Geometry check sheet. Reference: the model listing, model coordinates, mm. Face numbers are marked on the shaded views. A direction names the side the tool comes from. Round coordinates to 2 decimals unless told otherwise and drop trailing zeros. Write each loop counter-clockwise with the first axis right and the second up, starting at its lowest first coordinate (ties: lowest second). Pieces come first, ordered by that corner, then holes. Notation, with made-up numbers: M 33.5,37.5 L 46.5,37.5 A25 cw 46.5,65.5 Z; hole C 38,-36.75 d8. An arc over 180 degrees is marked long. Answer in a Markdown table with one row per item. Add a question column.
from build123d import *

# Parameters (mm, degrees)
EXTRUDE_1_DEPTH          = 0.75
PATTERN_CIRCULAR_1_COUNT = 14
SKETCH_3_W               = 6.1
SKETCH_3_H               = 6.1
EXTRUDE_2_DEPTH          = 9
FILLET_1_R               = 2
CHAMFER_1_SIZE           = 0.2
CHAMFER_1_SIZE2          = 2.286010461


with BuildPart() as part:
    # Sketch 1 → Revolve 1 (revolve)
    with BuildSketch(Plane(origin=(0, 0, 0), x_dir=(0, 0, -1), z_dir=(1, 0, 0)), mode=Mode.PRIVATE) as revolve_1_sk:
        Polygon((-5, 0), (5, 0), (5, 15), (3, 15), (3, 10), (-3, 10), (-3, 15), (-5, 15), align=None)
    revolve(revolve_1_sk.sketch.rotate(Axis((0, 0, 5), (0, 0, -1)), 90), axis=Axis((0, 0, 5), (0, 0, -1)))

    # Sketch 2 → Extrude 1 (add, symmetric)
    with BuildSketch(Plane(origin=(0, 0, 0), x_dir=(0, 0, -1), z_dir=(1, 0, 0))):
        with BuildLine():
            Line((3, 10), (3, 14))
            Line((3, 14), (2, 14))
            ThreePointArc((2, 14), (0, 12), (-2, 14))
            Line((-2, 14), (-3, 14))
            Line((-3, 14), (-3, 10))
            Line((-3, 10), (-3, 8.5))
            Line((-3, 8.5), (3, 8.5))
            Line((3, 8.5), (3, 10))
        make_face()
    extrude_1 = extrude(amount=EXTRUDE_1_DEPTH, both=True)

    # Pattern Circular 1: Extrude 1 ×14 about axis
    pattern_circular_1_axis = Axis((0, 0, 0), (0, 0, 1))
    for i in range(1, PATTERN_CIRCULAR_1_COUNT):
        add(extrude_1.rotate(pattern_circular_1_axis, i * 360 / PATTERN_CIRCULAR_1_COUNT))

    # Sketch 3 → Extrude 2 (add)
    with BuildSketch(Plane(origin=(0, 0, -5), x_dir=(-1, 0, 0), z_dir=(0, 0, -1))):
        with BuildLine():
            Line((-4.05, -6.05), (4.05, -6.05))
            ThreePointArc((4.05, -6.05), (5.464213562, -5.464213562), (6.05, -4.05))
            Line((6.05, -4.05), (6.05, 4.05))
            ThreePointArc((6.05, 4.05), (5.464213562, 5.464213562), (4.05, 6.05))
            Line((4.05, 6.05), (-4.05, 6.05))
            ThreePointArc((-4.05, 6.05), (-5.464213562, 5.464213562), (-6.05, 4.05))
            Line((-6.05, 4.05), (-6.05, -4.05))
            ThreePointArc((-6.05, -4.05), (-5.464213562, -5.464213562), (-4.05, -6.05))
        make_face()
        Rectangle(SKETCH_3_W, SKETCH_3_H, mode=Mode.SUBTRACT)
    extrude(amount=EXTRUDE_2_DEPTH)

    # Fillet 1
    fillet_1_edges = [part.edges().sort_by_distance(p)[0] for p in [
        (5.464213562, -5.464213562, -5),
        (0, -6.05, -5),
        (-5.464213562, -5.464213562, -5),
        (-6.05, 0, -5),
        (-5.464213562, 5.464213562, -5),
        (0, 6.05, -5),
        (5.464213562, 5.464213562, -5),
        (6.05, 0, -5),
    ]]
    fillet(fillet_1_edges, radius=FILLET_1_R)

    # Chamfer 1
    chamfer_1_edges = [part.edges().sort_by_distance(p)[0] for p in [
        (-3.05, 0, -14),
        (0, 3.05, -14),
        (3.05, 0, -14),
        (0, -3.05, -14),
    ]]
    chamfer_1_side = [part.faces().sort_by_distance(p)[0] for p in [
        (5.343213562, -5.343213562, -14),
    ]]
    chamfer(chamfer_1_edges, length=CHAMFER_1_SIZE, length2=CHAMFER_1_SIZE2, reference=chamfer_1_side[0])


solid = part.part
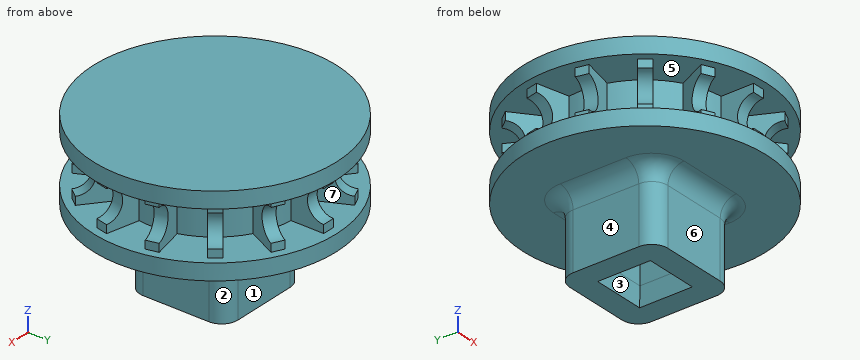
Item 1: Section check C-C, the plane z = 3.75. Record the boundary of the cut face in (x, y), and give its area (3 significant figures).
Item 2: Gauge pin test, flat ends, axial feed: pin 1 Ø0.8 at (x, z) = (0, 2.5) entering from +Y; pin 2 Ø1.8 at (y, z) = (1.5, -9.5) entering from +X; pin 3 Ø4.5 at (y, z) = (13, -0.5) entering from +X. Record the tip position at first contact, or that the pin passes through.
Item 3: Mould release check, pull along Y, two halves, no side actions. Record for the marked faces 5, 6 and 7: +Y half, -Y half, draft (parallel to the pull), parting line (faces both ways), or undercut.
Item 4: Section check B-B, the plane x = 0. Record the boundary of the cut face in (y, z).
Item 5: Access from +Z, -Z, +X, -X, +Y, -Y to the whole of each face (thin tool, end or side, straight path). Record for the marked faces 1, 2, 3 and 4.
Item 6: Scan lines: probe 1 along Z at (x, y) = (10.25, -3.5); probe 2 along Y at (x, z) = (-0.5, -4); probe 3 along X at (y, z) = (-0.75, -6.25). Record each from-to range of solid material in increasing order. Write a range as from..to.
Item 7: Section check A-A, the plane y = 0. Record the boundary of the cut face in (x, z), and give its area (3 significant figures).
Result sheet:
| question | item | result |
|---|---|---|
| 1 | outline | C 0,0 d30 |
| 1 | area | 707 mm^2 |
| 2 | pin 1 | stops at y = 14 |
| 2 | pin 2 | stops at x = 6.05 |
| 2 | pin 3 | stops at x = 6.75 |
| 3 | face 5 | undercut |
| 3 | face 6 | -Y half |
| 3 | face 7 | +Y half |
| 4 | outline | M -15,-5 L -8.05,-5 A2 cw -6.05,-7 L -6.05,-14 L -3.25,-14 L -3.05,-11.71 L -3.05,-5 L 3.05,-5 L 3.05,-11.71 L 3.25,-14 L 6.05,-14 L 6.05,-7 A2 cw 8.05,-5 L 15,-5 L 15,-3 L 14,-3 L 14,-2 A2 cw 14,2 L 14,3 L 15,3 L 15,5 L -15,5 L -15,3 L -14,3 L -14,2 A2 cw -14,-2 L -14,-3 L -15,-3 Z |
| 5 | face 1 | -Z, +X, -X, +Y |
| 5 | face 2 | -Z, +X, +Y |
| 5 | face 3 | -Z |
| 5 | face 4 | -Z, -X, +Y, -Y |
| 6 | probe 1 | z = -5..-3, 3..5 |
| 6 | probe 2 | y = -14.99..14.99 |
| 6 | probe 3 | x = -6.2..-3.05, 3.05..6.2 |
| 7 | outline | M -15,-5 L -8.05,-5 A2 cw -6.05,-7 L -6.05,-14 L -3.25,-14 L -3.05,-11.71 L -3.05,-5 L 3.05,-5 L 3.05,-11.71 L 3.25,-14 L 6.05,-14 L 6.05,-7 A2 cw 8.05,-5 L 15,-5 L 15,-3 L 10,-3 L 10,3 L 15,3 L 15,5 L -15,5 L -15,3 L -10,3 L -10,-3 L -15,-3 Z |
| 7 | area | 295 mm^2 |
